Here's how the part is built. I have some questions about the finished solid (model axes, mm). Face numbers are marked on the shaded views. Give positions to 0.01 mm unless a question says otherwise; leave off trailing zeros. Loops run counter-clockwise (first coordinate to the right, second up) from the corner with the lowest first, then second, coordinate; pieces in that order, holes last. Notation, with made-up numbers: (51.5, 5.25) - (86.5, 5.25) arc R23 cw to (86.5, 14.25) - close; hole circle Ø1 at (49.5, 13). An arc over 180 degrees is marked (long way). One line per item, written item: value. Start each with the question number.
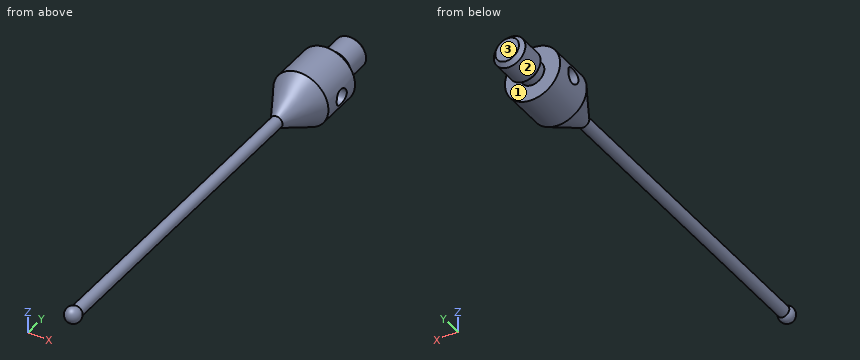
```python
from build123d import *

# Parameters (mm, degrees)
SKETCH2_R               = 0.75
BOSS_EXTRUDE2_DEPTH     = 40
SKETCH4_R               = 3.5
BOSS_EXTRUDE3_DEPTH     = 10
CHAMFER1_SIZE           = 4.763139721
CHAMFER1_SIZE_2         = 2.75
CUT_EXTRUDE4_DEPTH      = 51.244402673
CUT_EXTRUDE4_DEPTH_BACK = 51.244402673
SKETCH5_R               = 1
SKETCH6_R               = 1.5
BOSS_EXTRUDE4_DEPTH     = 1
SKETCH7_R               = 2
BOSS_EXTRUDE5_DEPTH     = 4
CHAMFER2_SIZE           = 0.5


# Some blends are built 0.0001 mm under size
with BuildPart() as part:
    # Sketch1 → Revolve1 (revolve)
    with BuildSketch(Plane.XY):
        with BuildLine():
            Line((0, 0), (0, -1))
            ThreePointArc((0, -1), (1, 0), (0, 1))
            Line((0, 1), (0, 0))
        make_face()
    revolve(axis=Axis((0, 0, 0), (0, 1, 0)))

    # Sketch2 → Boss-Extrude2 (add)
    with BuildSketch(Plane(origin=(0, 0, 0), x_dir=(1, 0, 0), z_dir=(0, 1, 0))):
        with Locations(Location((0, 0, 0), (0, 0, 90))):
            Circle(SKETCH2_R)
    extrude(amount=BOSS_EXTRUDE2_DEPTH)

    # Sketch4 → Boss-Extrude3 (add)
    with BuildSketch(Plane(origin=(0, 40, 0), x_dir=(1, 0, 0), z_dir=(0, 1, 0))):
        with Locations(Location((0, 0, 0), (0, 0, 270))):
            Circle(SKETCH4_R)
    extrude(amount=BOSS_EXTRUDE3_DEPTH)

    # Chamfer1
    # the kernel refuses this chamfer: 4.763139721, 2.75 mm, written as the material it takes off along each edge
    with BuildSketch(Plane(origin=(0, 40, 0), x_dir=(0, 0, 1), z_dir=(-1, 0, 0))) as chamfer1_piece_1_section:
        Polygon((3.5, CHAMFER1_SIZE), (3.5 - CHAMFER1_SIZE_2, 0), (3.5, 0), align=None)
    chamfer1_piece_1 = revolve(axis=Axis((0, 40, 0), (0, 1, 0)), mode=Mode.PRIVATE)
    chamfer1_piece_1 = chamfer1_piece_1 - Plane(origin=(0, 42.439255441, 0), x_dir=(0, 0, -1), z_dir=(0, -1, 0)) * Cylinder(0.75, 20, mode=Mode.PRIVATE)
    add(chamfer1_piece_1, mode=Mode.SUBTRACT)

    # Sketch5 → Cut-Extrude4 (cut, two sides: drawn at the far end of the back side and taken through both)
    with BuildSketch(Plane(origin=(0, 0, 0), x_dir=(0, 0, -1), z_dir=(1, 0, 0)).offset(-CUT_EXTRUDE4_DEPTH_BACK)):
        with Locations((0, 47.38156986)):
            Circle(SKETCH5_R)
    extrude(amount=CUT_EXTRUDE4_DEPTH + CUT_EXTRUDE4_DEPTH_BACK, mode=Mode.SUBTRACT)

    # Sketch6 → Boss-Extrude4 (add)
    with BuildSketch(Plane(origin=(0, 50, 0), x_dir=(1, 0, 0), z_dir=(0, 1, 0))):
        with Locations(Location((0, 0, 0), (0, 0, 270))):
            Circle(SKETCH6_R)
    extrude(amount=BOSS_EXTRUDE4_DEPTH)

    # Sketch7 → Boss-Extrude5 (add)
    with BuildSketch(Plane(origin=(0, 51, 0), x_dir=(1, 0, 0), z_dir=(0, 1, 0))):
        with Locations(Location((0, 0, 0), (0, 0, 270))):
            Circle(SKETCH7_R)
    extrude(amount=BOSS_EXTRUDE5_DEPTH)

    # Chamfer2
    chamfer2_edges = [part.edges().sort_by_distance(p)[0] for p in [
        (0, 51, -2),
        (0, 55, -2),
    ]]
    chamfer(chamfer2_edges, length=CHAMFER2_SIZE - 0.0001)  # a hair under: the kernel refuses the full size


solid = part.part
```
(1) Will these pins go through, and if not, where does the flat tip stop? pin 1 (1.5 mm diameter, centred on x = 0, z = -1, fed in from -Y); pin 2 (1 mm diameter, centred on x = 2, y = 31, fed in from +Z); pin 3 (2 mm diameter, centred on x = 2.5, z = -2, fed in from -Y).
(2) If we section it at A-A on y = 17.5: List the corners of the cut face in (x, z) for me, plus the area to 3 significant figures.
(3) Please list where these lines run through material, in increasing order: probe 1 along Y at (x, z) = (1.75, 0); probe 2 along Y at (x, z) = (1.25, 0); probe 3 along Y at (x, z) = (0.75, -1.75). Write a range as from..to.
(4) If we mould it in two halves opening along Y, with no side actions, what happens to the marked faces 1, 2 and 3? For each: pulls with the +Y half, pulls with the -Y half, needs draft (parallel to the pull), parting line crosses it, or undercut.
Found:
1. pin 1: y = -0.97
1. pin 2: through
1. pin 3: y = 42.51
2. outline: circle Ø1.5 at (0, 0)
2. area: 1.77 mm^2
3. probe 1: 41.73..46.38, 48.38..50, 51.25..54.75
3. probe 2: 40.87..46.38, 48.38..55
3. probe 3: 42..50, 51.4..54.6
4. face 1: undercut
4. face 2: needs draft
4. face 3: pulls with the +Y half
